```python
from build123d import *

# Parameters (mm, degrees)
F0_W     = 508
F0_H     = 508
F0_W_2   = 152.4
F0_H_2   = 152.4
F1_DEPTH = 863.6
F2_W     = 609.6
F2_H     = 609.6
F3_DEPTH = 50.8
F4_W     = 152.4
F4_H     = 152.4
F5_DEPTH = 254


with BuildPart() as f1:
    # F0 (on Top) → F1 (new body)
    with BuildSketch(Plane.XY):
        Rectangle(F0_W, F0_H)
        Rectangle(F0_W_2, F0_H_2, mode=Mode.SUBTRACT)
    extrude(amount=F1_DEPTH)

    # F2 (on face) → F3 (join)
    with BuildSketch(Plane.XY.offset(863.6)):
        Rectangle(F2_W, F2_H)
    extrude(amount=F3_DEPTH)

    # F4 (on face) → F5 (cut)
    with BuildSketch(Plane.XY.offset(914.4)):
        Rectangle(F4_W, F4_H)
    extrude(amount=-F5_DEPTH, mode=Mode.SUBTRACT)


solid = f1.part
```
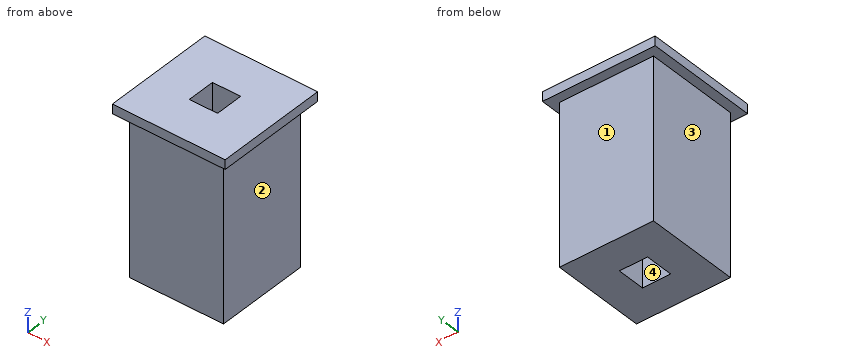
Can you work these out from the model? Positions are in its coordinate system, mm. Face numbers are marked on the shaded views. A direction names the side the tool comes from. Round coordinates to 2 decimals unless told otherwise and drop trailing zeros. Order: outer loops, then holes, each group sorted by start corner. A loop starts at its lowest first (then second) coordinate and runs counter-clockwise, first axis right, second up.
(1) If we section it at C-C (z = 829.5): Please give me the cut outline in (x, y), plus the area to 3 significant figures.
Results are:
outline: (-254, -254) - (254, -254) - (254, 254) - (-254, 254) - close; hole (-76.2, -76.2) - (76.2, -76.2) - (76.2, 76.2) - (-76.2, 76.2) - close
area: 235,000 mm2
(2) If I drill on L1, parallel to X at y = 63.5, z = 432; L2, parallel to Y at x = 118, z = 84, over which ranges is the centre line in solid material (lowest first)?
Results are:
L1: x = -254 to -76.2, 76.2 to 254
L2: y = -254 to 254
(3) If we section it at A-A (y = -27.5): Please give me the cut outline in (x, z).
Results are:
outline: (-304.8, 863.6) - (-254, 863.6) - (-254, 0) - (-76.2, 0) - (-76.2, 914.4) - (-304.8, 914.4) - close; (76.2, 0) - (254, 0) - (254, 863.6) - (304.8, 863.6) - (304.8, 914.4) - (76.2, 914.4) - close
(4) I'm going to push flat-ended pins straight in: pin 1 (12 mm diameter, centred on y = -171, z = 762.5, fed in from +X); pin 2 (5 mm diameter, centred on x = -61, z = 450, fed in from -Y); pin 3 (1 mm diameter, centred on x = -64.5, z = 371.5, fed in from +Y); pin 4 (12 mm diameter, centred on x = -65.5, y = 51, fed in from +Z). Where does each tip first touch, or does it pass through?
Results are:
pin 1: stops at x = 254
pin 2: stops at y = -254
pin 3: stops at y = 254
pin 4: passes through
(5) On a 3-axis mill with a long thin cutter (end or side, diameter ignored), from which of +Z, -Z, +X, -X, +Y, -Y can I reach the whole of each face in a straight line? I mean the marked faces 1, 2, 3 and 4. Say none if no direction works.
Results are:
face 1: -Z, +X, -X, +Y
face 2: -Z, +X, +Y, -Y
face 3: -Z, -X, +Y, -Y
face 4: +Z, -Z
(6) If we section it at D-D (x = 166.5): Please give me the cut outline in (y, z).
Results are:
outline: (-304.8, 863.6) - (-254, 863.6) - (-254, 0) - (254, 0) - (254, 863.6) - (304.8, 863.6) - (304.8, 914.4) - (-304.8, 914.4) - close
